Read the model definition and answer for the solid it produces. Units are mm, in the model's axes. Face numbers are marked on the shaded views. A direction names the side the tool comes from. Coordinates: 2 decimals unless noted, no trailing zeros. Order: outer loops, then holes, each group sorted by start corner. A loop starts at its lowest first (then second) coordinate and runs counter-clockwise, first axis right, second up. Notation, with made-up numbers: (-17, 74) -> (38, 74) arc R33 cw to (38, 102) -> close; hole circle Ø5 at (5.25, 78). An arc over 180 degrees is marked (long way). Answer as a JSON object with one key per item and string values. Group by question number.
1) Consider L1, parallel to X at y = 2.5, z = 0; L2, parallel to Y at x = 3.75, z = -9.5; L3, parallel to Z at x = 2.5, y = -13. Determine where each line is inside the solid, lowest interval first.
2) Section C-C on y = 1 is taken. Determine the outline of the cut face in (x, z).
3) Given pin 1 (1 mm diameter, centred on x = -3.5, y = 8, fed in from -Z); pin 2 (4 mm diameter, centred on x = -2, y = 10, fed in from +Z); pin 3 (6 mm diameter, centred on y = -9.5, z = -0.5, fed in from -X), each flat-ended and moving along its own axis, determine where each tip first touches the part or whether it passes through.
4) Section A-A on x = 0 is taken. Determine the outline of the cut face in (y, z).
5) A tool of negligible diameter and unlimited length cuts with its end or side. For the marked faces 4 and 5, from which of +Z, -Z, +X, -X, +Y, -Y can it reach the whole face along a straight path? Write none if from no direction.
6) Determine the mould class of the marked faces 1, 2 and 3 for opening direction Z: released by +Z, released by -Z, zero draft, split by the parting line, or undercut.
7) Section B-B on z = 0 is taken. Determine the outline of the cut face in (x, y).
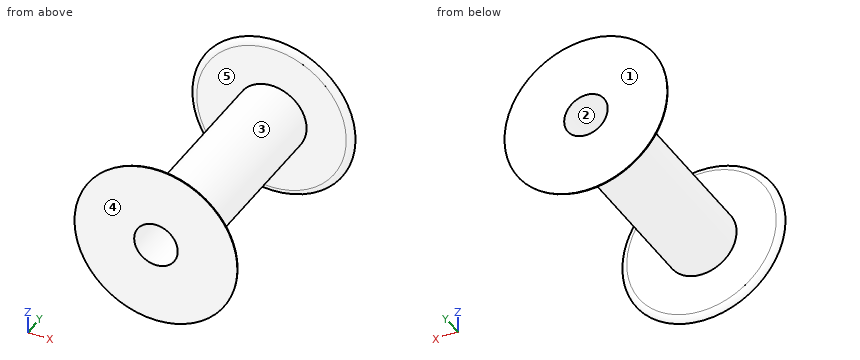
from build123d import *

# Parameters (mm, degrees)
SKETCH2_R          = 3.1
CUT_EXTRUDE1_DEPTH = 37.13806857
FILLET1_R          = 1


with BuildPart() as part:
    # Sketch1 → Revolve1 (revolve)
    with BuildSketch(Plane.XY, mode=Mode.PRIVATE) as revolve1_sk:
        Polygon((0, 0), (0, 16.1), (11.6, 16.1), (11.6, 15.4), (5, 15.4), (5, 0), align=None)
    revolve(revolve1_sk.sketch.rotate(Axis((0, 24.358616114, 0), (0, 1, 0)), 90), axis=Axis((0, 24.358616114, 0), (0, 1, 0)))

    # Mirror1: part across plane


with BuildPart() as part_1:
    add(part.part)
    add(part.part.mirror(Plane(origin=(5, 0, 0), x_dir=(0, 0, 1), z_dir=(0, -1, 0))))

    # Sketch2 → Cut-Extrude1 (cut, through all)
    with BuildSketch(Plane(origin=(0, 16.1, 0), x_dir=(1, 0, 0), z_dir=(0, 1, 0))):
        with Locations(Location((0, 0, 0), (0, 0, 270))):
            Circle(SKETCH2_R)
    extrude(amount=-CUT_EXTRUDE1_DEPTH, mode=Mode.SUBTRACT)

    # Fillet1
    # the kernel refuses this fillet: 1 mm, written as the material it takes off along each edge
    with BuildSketch(Plane(origin=(0, -15.4, 0), x_dir=(0, 0, -1), z_dir=(1, 0, 0))) as fillet1_piece_1:
        with BuildLine():
            CenterArc((10.646060799, -1), FILLET1_R, 17.457603124, 72.542396876)
            Line((10.646060799, 0), (10.646060799, 0.02))
            Line((10.646060799, 0.02), (11.6, 0.02))
            Line((11.6, 0.02), (11.62, 0))
            ThreePointArc((11.62, 0), (11.62, -0.35), (11.619078784, -0.694))
            Line((11.619078784, -0.694), (11.6, -0.7))
        make_face()
    revolve(axis=Axis((0, -15.4, 0), (0, 1, 0)), mode=Mode.SUBTRACT)
    with BuildSketch(Plane(origin=(0, 15.4, 0), x_dir=(0, 0, -1), z_dir=(1, 0, 0))) as fillet1_piece_2:
        with BuildLine():
            CenterArc((10.646060799, 1), FILLET1_R, 270, 72.542396876)
            Line((10.646060799, 0), (10.646060799, -0.02))
            Line((10.646060799, -0.02), (11.6, -0.02))
            Line((11.6, -0.02), (11.62, 0))
            ThreePointArc((11.62, 0), (11.62, 0.35), (11.619078784, 0.694))
            Line((11.619078784, 0.694), (11.6, 0.7))
        make_face()
    revolve(axis=Axis((0, 15.4, 0), (0, 1, 0)), mode=Mode.SUBTRACT)


solid = part_1.part
Worked answers:
{
 "1": {"L1": "x = -5 to -3.1, 3.1 to 5", "L2": "y = -16.1 to -15.4, 15.4 to 16.1", "L3": "z = -4.33 to -1.83, 1.83 to 4.33"},
 "2": {"outline": "circle Ø10 at (0, 0); hole circle Ø6.2 at (0, 0)"},
 "3": {"pin 1": "stops at z = -4", "pin 2": "stops at z = 5", "pin 3": "stops at x = -5"},
 "4": {"outline": "(-16.1, -11.6) arc R1 ccw to (-15.4, -10.65) -> (-15.4, -5) -> (15.4, -5) -> (15.4, -10.65) arc R1 ccw to (16.1, -11.6) -> (16.1, -3.1) -> (-16.1, -3.1) -> close; (-16.1, 3.1) -> (16.1, 3.1) -> (16.1, 11.6) arc R1 ccw to (15.4, 10.65) -> (15.4, 5) -> (-15.4, 5) -> (-15.4, 10.65) arc R1 ccw to (-16.1, 11.6) -> close"},
 "5": {"face 4": "+Z, -Z, +X, -X, -Y", "face 5": "none"},
 "6": {"face 1": "zero draft", "face 2": "undercut", "face 3": "split by the parting line"},
 "7": {"outline": "(-11.6, -16.1) -> (-3.1, -16.1) -> (-3.1, 16.1) -> (-11.6, 16.1) arc R1 ccw to (-10.65, 15.4) -> (-5, 15.4) -> (-5, -15.4) -> (-10.65, -15.4) arc R1 ccw to start; (3.1, -16.1) -> (11.6, -16.1) arc R1 ccw to (10.65, -15.4) -> (5, -15.4) -> (5, 15.4) -> (10.65, 15.4) arc R1 ccw to (11.6, 16.1) -> (3.1, 16.1) -> close"}
}
